```python
from build123d import *

# Parameters (mm, degrees)
SWEEP5_PROFILE_R         = 8
TAGLIO_ESTRUSIONE1_REACH = 114
SCHIZZO15_R              = 4


with BuildPart() as part:
    # Sweep5: sweep along a path in Schizzo1
    with BuildLine(Plane.XY) as sweep5_path:
        Line((-132.062548693, 77.708245302), (-212.062548693, 77.708245302))
        Line((-212.062548693, 77.708245302), (-212.062548693, -2.291754698))
        Line((-212.062548693, -2.291754698), (-132.062548693, -2.291754698))
        Line((-132.062548693, -2.291754698), (-132.062548693, 77.708245302))
    # Sweep5 profile (on start of the path) → Sweep5 (sweep)
    with BuildSketch(Plane(origin=(-132.062548693, 77.708245302, 0), x_dir=(0, -1, 0), z_dir=(-1, 0, 0))):
        Circle(SWEEP5_PROFILE_R)
    sweep(path=sweep5_path.line, transition=Transition.RIGHT)

    # Schizzo14 → Rivoluzione1 (revolve)
    with BuildSketch(Plane(origin=(-172.062548693, 0, 0), x_dir=(0, -1, 0), z_dir=(1, 0, 0))):
        with BuildLine():
            Line((-77.708245302, 0), (-101.708245302, 0))
            Line((-101.708245302, 0), (-101.708245302, 8))
            Line((-101.708245302, 8), (-109.708245302, 8))
            Line((-109.708245302, 8), (-109.708245302, 10))
            Line((-109.708245302, 10), (-97.708245302, 10))
            Line((-97.708245302, 10), (-97.708245302, 9.9))
            ThreePointArc((-97.708245302, 9.9), (-97.151748186, 8.556497116), (-95.808245302, 8))
            Line((-95.808245302, 8), (-77.708245302, 8))
            Line((-77.708245302, 8), (-77.708245302, 0))
        make_face()
    revolve(axis=Axis((-172.062548693, 29.552378968, 0), (0, 1, 0)))

    # Schizzo15 → Taglio-Estrusione1 (cut, up to next)
    with BuildSketch(Plane(origin=(0, 101.708245302, 0), x_dir=(1, 0, 0), z_dir=(0, 1, 0)), mode=Mode.PRIVATE) as taglio_estrusione1_sk1:
        with Locations((-172.062548693, 0)):
            Circle(SCHIZZO15_R)
    taglio_estrusione1_tool1 = extrude(taglio_estrusione1_sk1.sketch, amount=-TAGLIO_ESTRUSIONE1_REACH, mode=Mode.PRIVATE) & part.part
    add(taglio_estrusione1_tool1.solids().sort_by_distance((-172.062549, 101.708245, 0))[0], mode=Mode.SUBTRACT)


solid = part.part
```
Verification items for the finished model (mm, model axes). A direction names the side the tool comes from. Coordinates: 2 decimals unless noted, no trailing zeros. Write each loop counter-clockwise with the first axis right and the second up, starting at its lowest first coordinate (ties: lowest second). Pieces come first, ordered by that corner, then holes. Notation, with made-up numbers: M 49.25,-11.75 L 59.25,-11.75 A9 ccw 59.25,4.25 Z; hole C 78.5,-10 d9. An arc over 180 degrees is marked long. Answer as a JSON object with one key per item and string values. Group by question number.
(1) Material ranges on line 1 (X direction, y = 104.5, z = 0); line 2 (X direction, y = 91.5, z = 0); line 3 (Z direction, x = -181.5, y = 78), recorded low to high.
(2) Cross-section at D-D, the plane y = -1. Record the cut outline in (x, z).
(3) Cross-section at B-B, the plane y = 24. Record the cut outline in (x, z), and give its area (3 significant figures).
(4) Tool access check on faces 4 (the face through (-168.247, 85.932, -1.201)), 5 (the face through (-124.07, 38.38, 0.35)). Record the directions out of +Z, -Z, +X, -X, +Y, -Y that give a thin tool (end or side, any length) a straight path to the whole face; none if there is none.
(5) Cross-section at C-C, the plane y = 99.5. Record the cut outline in (x, z).
(6) Gauge pin test, flat ends, axial feed: pin 1 (1 mm diameter, centred on x = -181.5, z = -7, fed in from +Y); pin 2 (1.5 mm diameter, centred on y = 25, z = -3.5, fed in from -X); pin 3 (2 mm diameter, centred on x = -175, z = 2.5, fed in from +Y); pin 4 (6 mm diameter, centred on x = -181, y = 64, fed in from -Z). Record the tip position at first contact, or that the pin passes through.
(7) Release check for a two-part mould opening along X. For faces 1 (the face through (-180, 109.708, 3)), 2 (the face through (-164.965, 105.764, -3.692)), 3 (the face through (-180.49, 103.62, -5.38)) record: +X half, -X half, draft (parallel to the pull), parting line (faces both ways), or undercut.
(8) Cross-section at A-A, the plane z = 0. Record the cut outline in (x, y).
Reply:
{
 "1": {"line 1": "-182.06 to -180.06, -164.06 to -162.06", "line 2": "-180.06 to -176.06, -168.06 to -164.06", "line 3": "-7.99 to 7.99"},
 "2": {"outline": "M -210.77,-7.9 L -133.35,-7.9 A8 ccw long -133.35,7.9 L -210.77,7.9 A8 ccw long Z"},
 "3": {"outline": "C -212.06,0 d16; C -132.06,0 d16", "area": "402 mm²"},
 "4": {"face 4": "+Y", "face 5": "none"},
 "5": {"outline": "C -172.06,0 d20; hole C -172.06,0 d8"},
 "6": {"pin 1": "y = 82.37", "pin 2": "x = -219.58", "pin 3": "y = 101.71", "pin 4": "through"},
 "7": {"face 1": "draft", "face 2": "undercut", "face 3": "parting line"},
 "8": {"outline": "M -220.06,-10.29 L -124.06,-10.29 L -124.06,85.71 L -164.06,85.71 L -164.06,95.81 A1.9 cw -162.16,97.71 L -162.06,97.71 L -162.06,109.71 L -164.06,109.71 L -164.06,101.71 L -168.06,101.71 L -168.06,69.71 L -140.06,69.71 L -140.06,5.71 L -204.06,5.71 L -204.06,69.71 L -176.06,69.71 L -176.06,101.71 L -180.06,101.71 L -180.06,109.71 L -182.06,109.71 L -182.06,97.71 L -181.96,97.71 A1.9 cw -180.06,95.81 L -180.06,85.71 L -220.06,85.71 Z"}
}
